Input: dimensioned drawing with shaded views. Units: mm. Origin: part minimum x, y, z. Round coordinates to 2 decimals unless told otherwise and drop trailing zeros. Loops run counter-clockwise (first coordinate to the right, second up) from the corner with the lowest first, then second, coordinate; pieces in that order, holes last. Notation, with made-up numbers: M 31.25,-30 L 50.25,-30 A19 cw 50.25,-1 Z; hole C 62,17 d1. An arc over 180 degrees is marked long. Answer as a JSON object with one key per item and string values.
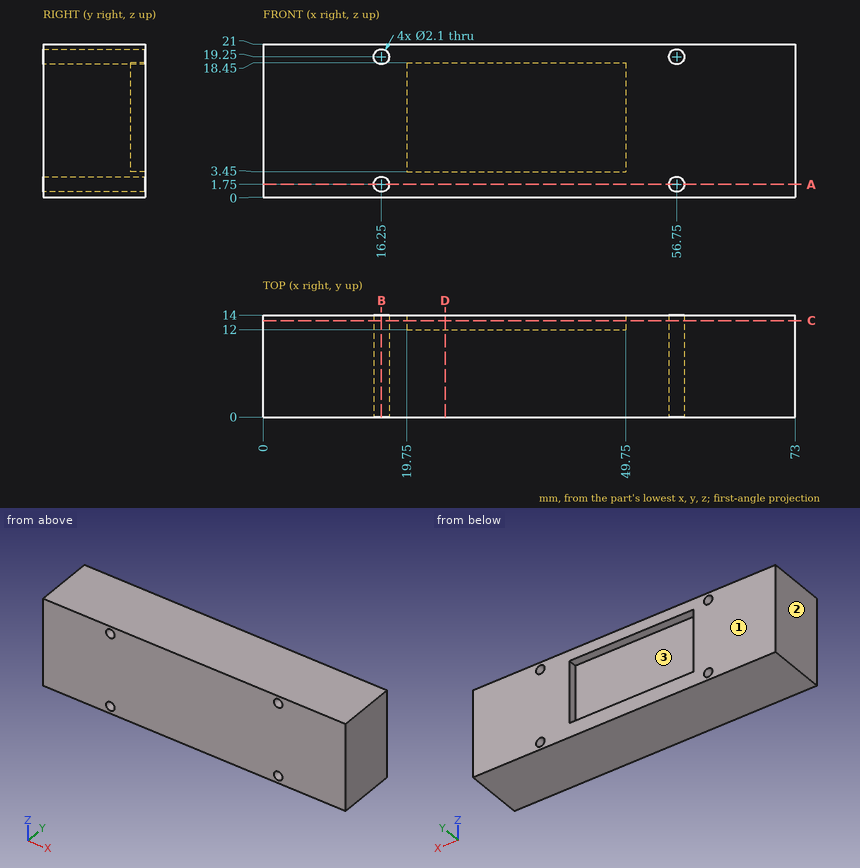
Item 1: Line query: probe 1 along X at (y, z) = (4, 1.75); probe 2 along X at (y, z) = (10.75, 2.5); probe 3 along Y at (x, z) = (41, 13.5). Output: solid intervals per line, ascending. Write a range as from..to.
Answer sheet:
{"probe 1": "x = 0..15.2, 17.3..55.7, 57.8..73", "probe 2": "x = 0..15.52, 16.98..56.02, 57.48..73", "probe 3": "y = 0..12"}
Item 2: Section A-A on z = 1.75. Return the cut outline in (x, y), then the cut area to 3 significant figures.
Answer sheet:
{"outline": "M 0,0 L 15.2,0 L 15.2,14 L 0,14 Z; M 17.3,0 L 55.7,0 L 55.7,14 L 17.3,14 Z; M 57.8,0 L 73,0 L 73,14 L 57.8,14 Z", "area": "963 mm²"}
Item 3: Section B-B on x = 16.25. Return the cut outline in (y, z).
Answer sheet:
{"outline": "M 0,0 L 14,0 L 14,0.7 L 0,0.7 Z; M 0,2.8 L 14,2.8 L 14,18.2 L 0,18.2 Z; M 0,20.3 L 14,20.3 L 14,21 L 0,21 Z"}
Item 4: Section D-D on x = 25. Return the cut outline in (y, z), then the cut area to 3 significant figures.
Answer sheet:
{"outline": "M 0,0 L 14,0 L 14,3.45 L 12,3.45 L 12,18.45 L 14,18.45 L 14,21 L 0,21 Z", "area": "264 mm²"}
Item 5: Contact query for flat-ended pins moving along their axis: pin 1 Ø1.9 at (x, z) = (16.25, 19.25) entering from +Y; pin 2 Ø2 at (x, z) = (46.5, 8.5) entering from +Y. Output: stop coordinate, or through.
Answer sheet:
{"pin 1": "passes through", "pin 2": "stops at y = 12"}
Item 6: Pull-direction query (X, two-part tool) for the marked faces 1, 2 and 3; classes: pulls with the +X half, pulls with the -X half, needs draft (parallel to the pull), parting line crosses it, or undercut.
Answer sheet:
{"face 1": "needs draft", "face 2": "pulls with the -X half", "face 3": "undercut"}
Item 7: Section C-C on y = 13.25. Return the cut outline in (x, z).
Answer sheet:
{"outline": "M 0,0 L 73,0 L 73,21 L 0,21 Z; hole C 16.25,1.75 d2.1; hole C 16.25,19.25 d2.1; hole M 19.75,3.45 L 49.75,3.45 L 49.75,18.45 L 19.75,18.45 Z; hole C 56.75,1.75 d2.1; hole C 56.75,19.25 d2.1"}
